from build123d import *

# Parameters (mm, degrees)
F0_W     = 266.7
F0_H     = 152.4
F0_R     = 19.05
F1_DEPTH = 50.8
F2_R     = 5.08


with BuildPart() as f1:
    # F0 (on Front) → F1 (new body)
    with BuildSketch(Plane.XZ):
        with Locations((-63.5, 0)):
            Circle(F0_R)
        with BuildLine():
            ThreePointArc((82.55, 0), (63.5, 19.05), (44.45, 0))
            ThreePointArc((44.45, 0), (63.5, -19.05), (82.55, 0))
        make_face()
        Rectangle(F0_W, F0_H)
        with Locations((-63.5, 0)):
            Circle(F0_R, mode=Mode.SUBTRACT)
        with BuildLine():
            ThreePointArc((-19.05, 0), (0, 19.05), (19.05, 0))
            ThreePointArc((19.05, 0), (0, -19.05), (-19.05, 0))
        make_face(mode=Mode.SUBTRACT)
        with BuildLine():
            ThreePointArc((82.55, 0), (63.5, -19.05), (44.45, 0))
            ThreePointArc((44.45, 0), (63.5, 19.05), (82.55, 0))
        make_face(mode=Mode.SUBTRACT)
    extrude(amount=F1_DEPTH)

    # F2
    f2_edges = [f1.edges().sort_by_distance(p)[0] for p in [
        (-133.35, -25.4, -76.2),
        (133.35, -25.4, -76.2),
        (0, 0, -76.2),
        (0, -50.8, -76.2),
        (133.35, -25.4, 76.2),
        (-133.35, -25.4, 76.2),
        (0, 0, 76.2),
        (0, -50.8, 76.2),
        (-133.35, 0, 0),
        (-133.35, -50.8, 0),
        (133.35, 0, 0),
        (133.35, -50.8, 0),
    ]]
    fillet(f2_edges, radius=F2_R)


solid = f1.part
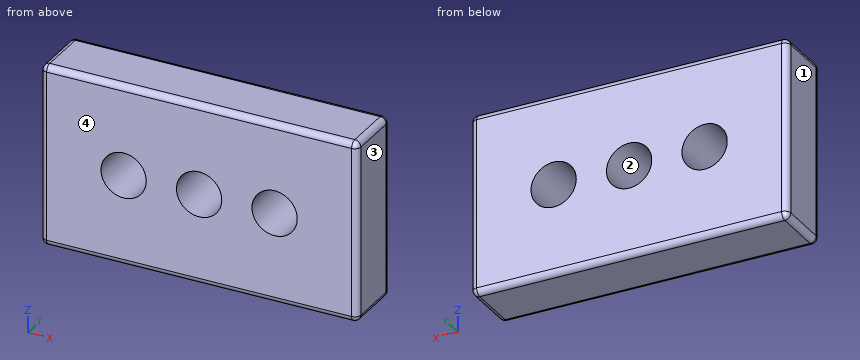
CAD build for the part. Positions are in the model's coordinates, mm. Face numbers are marked on the shaded views. Round coordinates to 2 decimals unless told otherwise and drop trailing zeros. Write each loop counter-clockwise with the first axis right and the second up, starting at its lowest first coordinate (ties: lowest second). Pieces come first, ordered by that corner, then holes. Notation, with made-up numbers: M 70.5,38.5 L 91.5,38.5 A30 ccw 91.5,65.5 Z; hole C 28.5,13 d3. An arc over 180 degrees is marked long. Put each result on its own line as item: value. Start each with the question number.
1) Drill centre lines: probe 1 along X at (y, z) = (-45.5, -5); probe 2 along Z at (x, y) = (-63.5, -18); probe 3 along Z at (x, y) = (-49, -37). Where is each one in solid material? Low to high. Write a range as [from, to].
2) Saw through at D-D, the plane x = -62.5. Write the cut outline in (y, z), and give its area (3 significant figures).
3) Saw through at C-C, the plane x = 63.5. Write the cut outline in (y, z), and give its area (3 significant figures).
4) Saw through at A-A, the plane y = -38. Write the cut outline in (x, z).
5) Pull direction X, two halves, no side cores. Call the marked faces 1, 2, 3 and 4: pulls with the +X half, pulls with the -X half, needs draft (parallel to the pull), parting line crosses it, or undercut.
6) Saw through at B-B, the plane z = 0. Write the cut outline in (x, y).
Resolved:
1. probe 1: [-133.35, -81.88], [-45.12, -18.38], [18.38, 45.12], [81.88, 133.35]
1. probe 2: [-76.2, -19.05], [19.05, 76.2]
1. probe 3: [-76.2, -12.36], [12.36, 76.2]
2. outline: M -50.8,-71.12 A5.08 ccw -45.72,-76.2 L -5.08,-76.2 A5.08 ccw 0,-71.12 L 0,-19.02 L -50.8,-19.02 Z; M -50.8,19.02 L 0,19.02 L 0,71.12 A5.08 ccw -5.08,76.2 L -45.72,76.2 A5.08 ccw -50.8,71.12 Z
2. area: 5,790 mm²
3. outline: M -50.8,-71.12 A5.08 ccw -45.72,-76.2 L -5.08,-76.2 A5.08 ccw 0,-71.12 L 0,-19.05 L -50.8,-19.05 Z; M -50.8,19.05 L 0,19.05 L 0,71.12 A5.08 ccw -5.08,76.2 L -45.72,76.2 A5.08 ccw -50.8,71.12 Z
3. area: 5,780 mm²
4. outline: M -133.35,-71.12 A5.08 ccw -128.27,-76.2 L 128.27,-76.2 A5.08 ccw 133.35,-71.12 L 133.35,71.12 A5.08 ccw 128.27,76.2 L -128.27,76.2 A5.08 ccw -133.35,71.12 Z; hole C -63.5,0 d38.1; hole C 0,0 d38.1; hole C 63.5,0 d38.1
5. face 1: pulls with the -X half
5. face 2: undercut
5. face 3: pulls with the +X half
5. face 4: needs draft
6. outline: M -133.35,-45.72 A5.08 ccw -128.27,-50.8 L -82.55,-50.8 L -82.55,0 L -128.27,0 A5.08 ccw -133.35,-5.08 Z; M -44.45,-50.8 L -19.05,-50.8 L -19.05,0 L -44.45,0 Z; M 19.05,-50.8 L 44.45,-50.8 L 44.45,0 L 19.05,0 Z; M 82.55,-50.8 L 128.27,-50.8 A5.08 ccw 133.35,-45.72 L 133.35,-5.08 A5.08 ccw 128.27,0 L 82.55,0 Z
